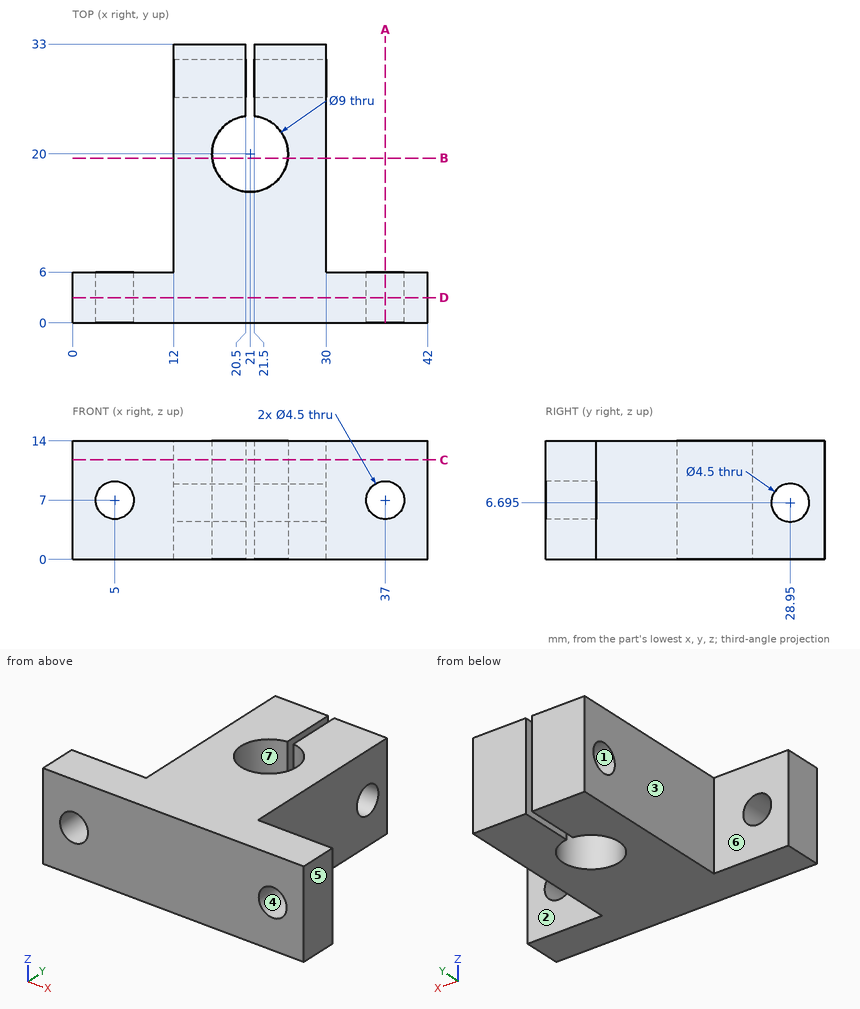
Job drawing, mm, ordinate dimensions from the low corner. One solid piece. A direction names the side the tool comes from. Round coordinates to 2 decimals unless told otherwise and drop trailing zeros. Loops run counter-clockwise (first coordinate to the right, second up) from the corner with the lowest first, then second, coordinate; pieces in that order, holes last. Notation, with made-up numbers: (83.25, 15.25) -> (100.25, 15.25) arc R10 cw to (100.25, 27.25) -> close; hole circle Ø8 at (-33.75, 48). An arc over 180 degrees is marked (long way). Use a Markdown table: item, result.
1) Cut at A-A, the plane x = 37. List the corners of the cut face in (y, z), and give its area (3 significant figures).
The answers:
| item | result |
|---|---|
| outline | (0, 0) -> (6, 0) -> (6, 4.75) -> (0, 4.75) -> close; (0, 9.25) -> (6, 9.25) -> (6, 14) -> (0, 14) -> close |
| area | 57.0 mm2 |
2) Tool access for the marked faces 1, 2 and 3: list every direction of +Z, -Z, +X, -X, +Y, -Y with a clear straight run to the whole face (end or side of a thin tool).
The answers:
| item | result |
|---|---|
| face 1 | +X, -X |
| face 2 | +Z, -Z, +X, +Y |
| face 3 | +Z, -Z, -X, +Y |
3) Cut at D-D, the plane y = 3. List the corners of the cut face in (x, z), and give its area (3 significant figures).
The answers:
| item | result |
|---|---|
| outline | (0, 0) -> (42, 0) -> (42, 14) -> (0, 14) -> close; hole circle Ø4.5 at (5, 7); hole circle Ø4.5 at (37, 7) |
| area | 556 mm2 |
4) Cut at C-C, the plane z = 11.75. List the corners of the cut face in (x, y).
The answers:
| item | result |
|---|---|
| outline | (0, 0) -> (42, 0) -> (42, 6) -> (30, 6) -> (30, 33) -> (21.5, 33) -> (21.5, 24.47) arc R4.5 cw (long way) to (20.5, 24.47) -> (20.5, 33) -> (12, 33) -> (12, 6) -> (0, 6) -> close |
5) Drop flat-ended pins along their axis: pin 1 Ø7 at (x, z) = (37, 7) entering from -Y; pin 2 Ø3 at (y, z) = (23.5, 8.5) entering from +X; pin 3 Ø6 at (y, z) = (28.95, 6.7) entering from -X; pin 4 Ø4 at (x, z) = (37, 3.5) entering from +Y. Give the stop position or say it passes through.
The answers:
| item | result |
|---|---|
| pin 1 | stops at y = 0 |
| pin 2 | stops at x = 30 |
| pin 3 | stops at x = 12 |
| pin 4 | stops at y = 6 |
6) Cut at B-B, the plane y = 19.5. List the corners of the cut face in (x, z), and give its area (3 significant figures).
The answers:
| item | result |
|---|---|
| outline | (12, 0) -> (16.53, 0) -> (16.53, 14) -> (12, 14) -> close; (25.47, 0) -> (30, 0) -> (30, 14) -> (25.47, 14) -> close |
| area | 127 mm2 |
7) Probe line 1 (X direction, y = 4.15, z = 7); line 2 (X direction, y = 29, z = 11.25); line 3 (Y direction, x = 17, z = 7.5). List the from-to ranges inside material, lowest first. Write a range as [from, to].
The answers:
| item | result |
|---|---|
| line 1 | x = [0, 2.75], [7.25, 34.75], [39.25, 42] |
| line 2 | x = [12, 20.5], [21.5, 30] |
| line 3 | y = [0, 17.94], [22.06, 26.85], [31.05, 33] |
8) Pull direction X, two halves, no side cores. Call the marked faces 4, 5, 6 and 7: pulls with the +X half, pulls with the -X half, needs draft (parallel to the pull), parting line crosses it, or undercut.
The answers:
| item | result |
|---|---|
| face 4 | undercut |
| face 5 | pulls with the +X half |
| face 6 | needs draft |
| face 7 | undercut |
